from build123d import *

# Parameters (mm, degrees)
SKETCH019_R             = 6.5
SKETCH019_R_2           = 2.5
PAD010_DEPTH            = 6
SKETCH020_R             = 5
SKETCH020_R_2           = 2.522437
PAD011_DEPTH            = 7
SKETCH021_R             = 6.5
SKETCH021_R_2           = 2.522437
PAD012_DEPTH            = 1
SKETCH022_R             = 1
PAD013_DEPTH            = 7
BODY011_PLACEMENT_ANGLE = 180


with BuildPart() as part:
    # Sketch019 → Pad010 (new body)
    with BuildSketch(Plane.YZ):
        Circle(SKETCH019_R)
        Circle(SKETCH019_R_2, mode=Mode.SUBTRACT)
    extrude(amount=PAD010_DEPTH)

    # Sketch020 (on Face3 of Pad010) → Pad011 (join)
    with BuildSketch(Plane(origin=(0, 0, 0), x_dir=(0, 1, 0), z_dir=(-1, 0, 0))):
        Circle(SKETCH020_R)
        Circle(SKETCH020_R_2, mode=Mode.SUBTRACT)
    extrude(amount=PAD011_DEPTH)

    # Sketch021 (on Face6 of Pad011) → Pad012 (join)
    with BuildSketch(Plane(origin=(-7, 0, 0), x_dir=(0, 1, 0), z_dir=(-1, 0, 0))):
        Circle(SKETCH021_R)
        Circle(SKETCH021_R_2, mode=Mode.SUBTRACT)
    extrude(amount=PAD012_DEPTH)

    # Sketch022 → Pad013 (join)
    with BuildSketch(Plane.XZ):
        with Locations((3, 0)):
            Circle(SKETCH022_R)
    extrude(amount=PAD013_DEPTH)


with BuildPart() as part_1:
    # Body011 placement: moved
    add(part.part.moved(Location((31, 0, 0))).rotate(Axis((31, 0, 0), (0, 0, 1)), BODY011_PLACEMENT_ANGLE))


solid = part_1.part
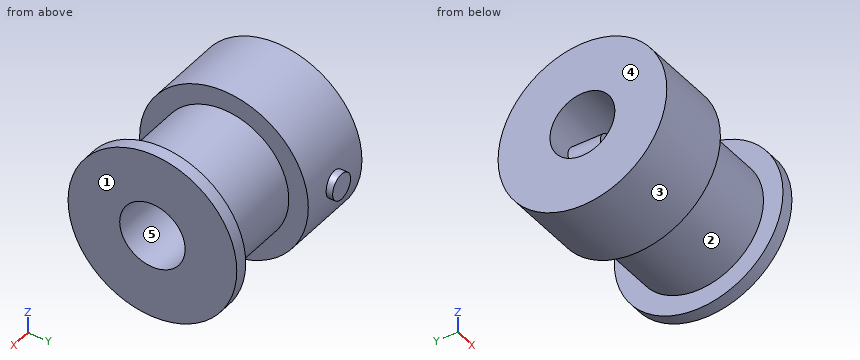
The listing builds one solid part. Answer for the finished solid, in the listing's coordinates (mm). Face numbers are marked on the shaded views. A direction names the side the tool comes from. Give positions to 0.01 mm unless a question says otherwise; leave off trailing zeros. Write each loop counter-clockwise with the first axis right and the second up, starting at its lowest first coordinate (ties: lowest second). Pieces come first, ordered by that corner, then holes.
1) For a pull along Z with two mould halves and no side action, classify the marked faces 3, 4 and 5 as pulls with the +Z half, pulls with the -Z half, needs draft (parallel to the pull), parting line crosses it, or undercut.
2) Given P1, Ø6, axis at x = 28.5, z = 4, coming from the -Y side; P2, Ø4, axis at x = 35, y = -4.5, coming from the +Z side; P3, Ø4, axis at y = 0, z = 0, coming from the -X side, each flat-ended and moving along its own axis, determine where each tip first touches the part or whether it passes through.
3) Section D-D (y = 4) is taken. Write down the section's boundary in (x, z).
4) Section C-C (x = 26.25) is taken. Write down the section's boundary in (y, z), and give its area (3 significant figures).
5) A tool of negligible diameter and unlimited length cuts with its end or side. For the marked faces 1 and 2, from which of +Z, -Z, +X, -X, +Y, -Y can it reach the whole face along a straight path? Write none if from no direction.
6) Section B-B (y = 5.75) is taken. Write down the section's boundary in (x, z), and give its area (3 significant figures).
7) Find the intervals of material crossed by L1, parallel to X at y = -0.5, z = 5.5; L2, parallel to Y at x = 29.25, z = 0; L3, parallel to Y at x = 28.75, z = 0, in increasing order.
Response:
1. face 3: parting line crosses it
1. face 4: needs draft
1. face 5: undercut
2. P1: stops at y = -6.42
2. P2: stops at z = 4.33
2. P3: stops at x = 27
3. outline: (25, -5.12) - (31, -5.12) - (31, -3) - (38, -3) - (38, -5.12) - (39, -5.12) - (39, 5.12) - (38, 5.12) - (38, 3) - (31, 3) - (31, 5.12) - (25, 5.12) - close
4. outline: circle Ø13 at (0, 0); hole circle Ø5 at (0, 0)
4. area: 113 mm2
5. face 1: +Z, -Z, +X, +Y, -Y
5. face 2: none
6. outline: (25, -3.03) - (31, -3.03) - (31, 3.03) - (25, 3.03) - close; (38, -3.03) - (39, -3.03) - (39, 3.03) - (38, 3.03) - close
6. area: 42.4 mm2
7. L1: x = 25 to 31, 38 to 39
7. L2: y = -6.5 to -2.5, 2.5 to 6.5
7. L3: y = -6.5 to -2.5, 0 to 7
